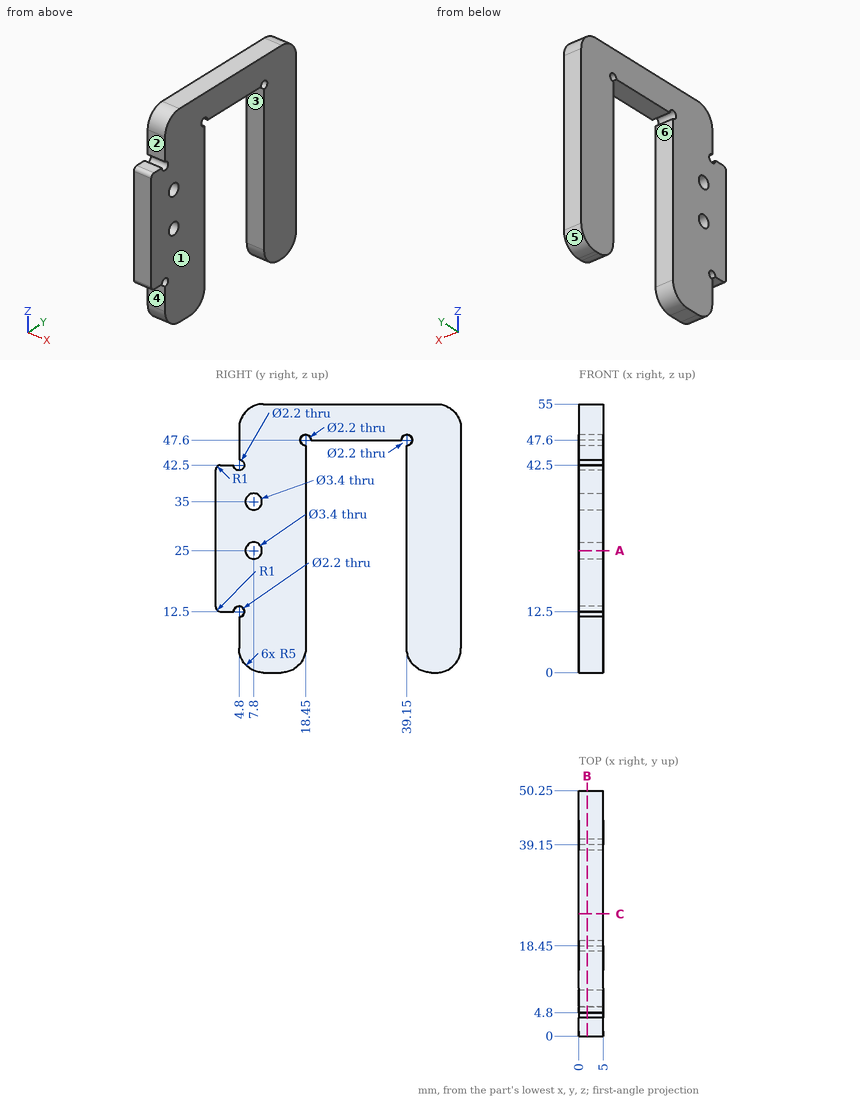
The figure shows three views and two pictorial views of one solid part (mm, origin at its lowest corner). Answer the questions. A direction names the side the tool comes from. Give positions to 0.01 mm unless a question says otherwise; leave off trailing zeros. Order: outer loops, then holes, each group sorted by start corner. A loop starts at its lowest first (then second) coordinate and runs counter-clockwise, first axis right, second up. Notation, with made-up numbers: (-6.5, 63.25) - (21.5, 63.25) arc R13 ccw to (21.5, 79.25) - close; hole circle Ø8 at (8.5, -15). An arc over 180 degrees is marked (long way). Answer as CSV lines item,"result".
Q1. Which of the six approach directions +Z, -Z, +X, -X, +Y, -Y give full straight-line access (tool end or side, diameter ignored) to the marked faces 1, 2 and 3?
Answer key:
face 1,"+Z, -Z, +X, +Y, -Y"
face 2,"+Z, +X, -X, -Y"
face 3,"-Z, +X, -X"
Q2. A cutting plane is placed at C-C, the plane y = 25. Determine the outline of the cut face in (x, z), and give its area (3 significant figures).
Answer key:
outline,"(0, 47.6) - (5, 47.6) - (5, 55) - (0, 55) - close"
area,"37.0 mm^2"
Q3. Straight lines are drawn through the part: L1, parallel to Y at x = 3.5, z = 25; L2, parallel to Y at x = 2.95, z = 9; L3, parallel to Z at x = 1, y = 5.5. For each, find the intervals that lie inside material, in ascending order.
Answer key:
L1,"y = 0 to 6.1, 9.5 to 18.45, 39.15 to 50.25"
L2,"y = 4.8 to 18.45, 39.15 to 50.25"
L3,"z = 2.45 to 11.65, 13.35 to 41.65, 43.35 to 52.55"
Q4. Each of these flat-tipped pins is pushed along its axis until it touches: pin 1 Ø3 at (x, y) = (2.5, 3) entering from +Z; pin 2 Ø1.5 at (x, z) = (3.5, 8.5) entering from -Y; pin 3 Ø2 at (x, y) = (2, 2) entering from -Z. Where does it stop, or does it pass through?
Answer key:
pin 1,"stops at z = 42.5"
pin 2,"stops at y = 4.8"
pin 3,"stops at z = 12.5"
Q5. A cutting plane is placed at B-B, the plane x = 1.65. Determine the outline of the cut face in (y, z), and give its area (3 significant figures).
Answer key:
outline,"(0, 13.5) arc R1 ccw to (1, 12.5) - (3.7, 12.5) arc R1.1 cw (long way) to (4.8, 11.4) - (4.8, 5) arc R5 ccw to (9.8, 0) - (13.45, 0) arc R5 ccw to (18.45, 5) - (18.45, 46.5) arc R1.1 cw (long way) to (19.55, 47.6) - (38.05, 47.6) arc R1.1 cw (long way) to (39.15, 46.5) - (39.15, 5) arc R5 ccw to (44.15, 0) - (45.25, 0) arc R5 ccw to (50.25, 5) - (50.25, 50) arc R5 ccw to (45.25, 55) - (9.8, 55) arc R5 ccw to (4.8, 50) - (4.8, 43.6) arc R1.1 cw (long way) to (3.7, 42.5) - (1, 42.5) arc R1 ccw to (0, 41.5) - close; hole circle Ø3.4 at (7.8, 25); hole circle Ø3.4 at (7.8, 35)"
area,"1,600 mm^2"
Q6. A cutting plane is placed at A-A, the plane z = 25. Determine the outline of the cut face in (x, y), and give its area (3 significant figures).
Answer key:
outline,"(0, 0) - (5, 0) - (5, 6.1) - (0, 6.1) - close; (0, 9.5) - (5, 9.5) - (5, 18.45) - (0, 18.45) - close; (0, 39.15) - (5, 39.15) - (5, 50.25) - (0, 50.25) - close"
area,"131 mm^2"
Q7. Determine the mould class of the marked faces 4, 5 and 6 for opening direction Y: pulls with the +Y half, pulls with the -Y half, needs draft (parallel to the pull), parting line crosses it, or undercut.
Answer key:
face 4,"pulls with the -Y half"
face 5,"pulls with the +Y half"
face 6,"undercut"
